from build123d import *

# Parameters (mm, degrees)
CIRPATTERN1_COUNT = 4
SKETCH4_W         = 3.7
SKETCH4_H         = 1.9


with BuildPart() as part:
    # Sketch2 → Revolve2 (revolve)
    with BuildSketch(Plane(origin=(0, 0, 0), x_dir=(1, 0, 0), z_dir=(0, 1, 0)), mode=Mode.PRIVATE) as revolve2_sk:
        Polygon((-15.340606893, 4), (-4.760755316, 4), (-0.364516129, 1.95), (1.635483871, 1.95), (9.659393107, 4.1), (9.659393107, 12.35), (-15.340606893, 12.35), align=None)
    revolve(revolve2_sk.sketch.rotate(Axis((-6.793548387, 0, 0), (1, 0, 0)), 180), axis=Axis((-6.793548387, 0, 0), (1, 0, 0)))

    # Sketch3 → M4x0.7 Tapped Hole1 (revolve, cut)
    with BuildSketch(Plane(origin=(-0.340606893, 11.787719099, 3.684043761), x_dir=(0, -0.2983031385746438, 0.9544711821299358), z_dir=(1, 0, 0))):
        Polygon((0, 0), (0, 7.991420021), (1.65, 7), (1.65, 0.85), (2.5, 0), align=None)
    m4x0_7_tapped_hole1 = revolve(axis=Axis((-0.340606893, 17.848611106, 5.578268691), (0, -0.9544711821299356, -0.2983031385746438)), mode=Mode.SUBTRACT)

    # CirPattern1: M4x0.7 Tapped Hole1 ×4 about axis
    cirpattern1_axis = Axis((-6.793548387, 0, 0), (-1, 0, 0))
    for i in range(1, CIRPATTERN1_COUNT):
        add(m4x0_7_tapped_hole1.rotate(cirpattern1_axis, i * 360 / CIRPATTERN1_COUNT), mode=Mode.SUBTRACT)

    # Sketch4 → Cut-Revolve1 (revolve, cut)
    with BuildSketch(Plane(origin=(0, 0, 0), x_dir=(1, 0, 0), z_dir=(0, 1, 0)), mode=Mode.PRIVATE) as cut_revolve1_sk:
        with Locations((-8.490606893, 11.4)):
            Rectangle(SKETCH4_W, SKETCH4_H)
    revolve(cut_revolve1_sk.sketch.rotate(Axis((-15.340606893, 0, 0), (1, 0, 0)), 180), axis=Axis((-15.340606893, 0, 0), (1, 0, 0)), mode=Mode.SUBTRACT)


solid = part.part
Verification items for the finished model (mm, model axes). A direction names the side the tool comes from. Coordinates: 2 decimals unless noted, no trailing zeros. Put each result on its own line as item: value. Start each with the question number.
1. Mould release check, pull along Z, two halves, no side actions. Record for faces 4 (the cylindrical face through (-12.88, -3.71, 11.78)), 5 (the flat face through (-15.341, -3, -3)), 6 (the conical face through (-0.231, -1.604, 4.246)): released by +Z, released by -Z, zero draft, split by the parting line, or undercut.
2. Material ranges on L1, parallel to Y at x = -10.5, z = 0; L2, parallel to Y at x = -8.5, z = 0; L3, parallel to X at y = -9.75, z = -2, recorded low to high. Write a range as [from, to].
3. Go/stop test with flat-tipped pins: pin 1 Ø2 at (x, z) = (-4, -7) entering from +Y; pin 2 Ø4 at (x, y) = (-0.5, -6.5) entering from -Z; pin 3 Ø2 at (x, z) = (0, -3.5) entering from +Y. Record where each tip stops, or that it passes through.
4. Access from +Z, -Z, +X, -X, +Y, -Y to the whole of each face (thin tool, end or side, straight path). Record for faces 1 (the cylindrical face through (1.4, -0.54, -12.34)), 2 (the cylindrical face through (-9.977, 3.905, -0.867)), 3 (the conical face through (-0.231, -4.246, -1.604)).
Computed:
1. face 4: split by the parting line
1. face 5: zero draft
1. face 6: undercut
2. L1: [-12.35, -4], [4, 12.35]
2. L2: [-10.45, -4], [4, 10.45]
2. L3: [-15.34, -1.65], [0.97, 9.66]
3. pin 1: y = 10.79
3. pin 2: z = -11.5
3. pin 3: y = 12.09
4. face 1: +X, -X
4. face 2: -X
4. face 3: none
